from build123d import *

# Parameters (mm, degrees)
EXTRUDE_1_DEPTH          = 32
SKETCH_3_R               = 40
CUT_EXTRUDE_1_DEPTH      = 12
SKETCH_4_R               = 32.5
CUT_EXTRUDE_2_DEPTH      = 113
SKETCH_5_R               = 23.5
CUT_EXTRUDE_3_DEPTH      = 13
SKETCH_6_R               = 21
CUT_EXTRUDE_4_DEPTH      = 113
SKETCH_7_R               = 22.5
CUT_EXTRUDE_5_DEPTH      = 40
SKETCH_8_R               = 41.5
CUT_EXTRUDE_6_DEPTH      = 5.5
SKETCH_9_R               = 31
CUT_EXTRUDE_7_DEPTH      = 10
SKETCH_10_R              = 2.5
CUT_EXTRUDE_8_DEPTH      = 18
PATTERN_CIRCULAR_1_COUNT = 4
SKETCH_12_W              = 185
SKETCH_12_H              = 5
CUT_EXTRUDE_10_DEPTH     = 114
SKETCH_13_R              = 6
CUT_EXTRUDE_11_DEPTH     = 14
SKETCH_14_R              = 4
SKETCH_14_R_2            = 4.76
CUT_EXTRUDE_12_DEPTH     = 96
SKETCH_15_R              = 7
CUT_EXTRUDE_13_DEPTH     = 9
SKETCH_16_R              = 2.531047244
SKETCH_16_R_2            = 3
CUT_EXTRUDE_14_DEPTH     = 10
SKETCH_17_R              = 2.5
CUT_EXTRUDE_15_DEPTH     = 8


with BuildPart() as part:
    # 草图1 → 凸台-拉伸1 (new body)
    with BuildSketch(Plane.XY):
        Polygon((105, -80), (105, -6), (150, -6), (150, 147), (-30, 147), (-80, 97), (-80, -80), align=None)
    extrude(amount=EXTRUDE_1_DEPTH)

    # 草图3 → 切除-拉伸1 (cut)
    with BuildSketch(Plane.XY.offset(32)):
        Circle(SKETCH_3_R)
    extrude(amount=-CUT_EXTRUDE_1_DEPTH, mode=Mode.SUBTRACT)

    # 草图4 → 切除-拉伸2 (cut)
    with BuildSketch(Plane.XY.offset(20)):
        Circle(SKETCH_4_R)
    extrude(amount=-CUT_EXTRUDE_2_DEPTH, mode=Mode.SUBTRACT)

    # 草图5 → 切除-拉伸3 (cut)
    with BuildSketch(Plane(origin=(0, 0, 0), x_dir=(-1, 0, 0), z_dir=(0, 0, -1))):
        with Locations((0, 85)):
            Circle(SKETCH_5_R)
    extrude(amount=-CUT_EXTRUDE_3_DEPTH, mode=Mode.SUBTRACT)

    # 草图6 → 切除-拉伸4 (cut)
    with BuildSketch(Plane(origin=(0, 0, 13), x_dir=(-1, 0, 0), z_dir=(0, 0, -1))):
        with Locations((0, 85)):
            Circle(SKETCH_6_R)
    extrude(amount=-CUT_EXTRUDE_4_DEPTH, mode=Mode.SUBTRACT)

    # 草图7 → 切除-拉伸5 (cut)
    with BuildSketch(Plane(origin=(0, 0, 0), x_dir=(-1, 0, 0), z_dir=(0, 0, -1))):
        with Locations((-80, 85)):
            Circle(SKETCH_7_R)
    extrude(amount=-CUT_EXTRUDE_5_DEPTH, mode=Mode.SUBTRACT)

    # 草图8 → 切除-拉伸6 (cut)
    with BuildSketch(Plane.XY.offset(32)):
        with Locations((80, 85)):
            Circle(SKETCH_8_R)
    extrude(amount=-CUT_EXTRUDE_6_DEPTH, mode=Mode.SUBTRACT)

    # 草图9 → 切除-拉伸7 (cut)
    with BuildSketch(Plane(origin=(0, 0, 0), x_dir=(-1, 0, 0), z_dir=(0, 0, -1))):
        with Locations((-80, 85)):
            Circle(SKETCH_9_R)
    extrude(amount=-CUT_EXTRUDE_7_DEPTH, mode=Mode.SUBTRACT)

    # 草图10 → 切除-拉伸8 (cut)
    with BuildSketch(Plane(origin=(0, 0, 0), x_dir=(-1, 0, 0), z_dir=(0, 0, -1))):
        with Locations((-41, 85)):
            Circle(SKETCH_10_R)
    cut_extrude_8 = extrude(amount=-CUT_EXTRUDE_8_DEPTH, mode=Mode.SUBTRACT)

    # 阵列(圆周)1: 切除-拉伸8 ×4 about axis
    pattern_circular_1_axis = Axis((80, 85, 0), (0, 0, 1))
    for i in range(1, PATTERN_CIRCULAR_1_COUNT):
        add(cut_extrude_8.rotate(pattern_circular_1_axis, i * 360 / PATTERN_CIRCULAR_1_COUNT), mode=Mode.SUBTRACT)

    # 草图12 → 切除-拉伸10 (cut)
    with BuildSketch(Plane(origin=(0, 0, 0), x_dir=(-1, 0, 0), z_dir=(0, 0, -1))):
        with Locations((-12.5, -77.5)):
            Rectangle(SKETCH_12_W, SKETCH_12_H)
    extrude(amount=-CUT_EXTRUDE_10_DEPTH, mode=Mode.SUBTRACT)

    # 草图13 → 切除-拉伸11 (cut)
    with BuildSketch(Plane.XY.offset(32)):
        with Locations((80, 34)):
            Circle(SKETCH_13_R)
        with Locations((80, 136)):
            Circle(SKETCH_13_R)
    extrude(amount=-CUT_EXTRUDE_11_DEPTH, mode=Mode.SUBTRACT)

    # 草图14 → 切除-拉伸12 (cut)
    with BuildSketch(Plane.XY.offset(32)):
        with Locations((140, 137)):
            Circle(SKETCH_14_R)
        with Locations((140, 4)):
            Circle(SKETCH_14_R_2)
        with Locations((32, 137)):
            Circle(SKETCH_14_R_2)
        with Locations((-70, -65)):
            Circle(SKETCH_14_R)
        with Locations((95, -65)):
            Circle(SKETCH_14_R)
        with Locations((-70, 87)):
            Circle(SKETCH_14_R)
    extrude(amount=-CUT_EXTRUDE_12_DEPTH, mode=Mode.SUBTRACT)

    # 草图15 → 切除-拉伸13 (cut)
    with BuildSketch(Plane.XY.offset(32)):
        with Locations((140, 137)):
            Circle(SKETCH_15_R)
        with Locations((95, -65)):
            Circle(SKETCH_15_R)
        with Locations((-70, -65)):
            Circle(SKETCH_15_R)
        with Locations((-70, 87)):
            Circle(SKETCH_15_R)
    extrude(amount=-CUT_EXTRUDE_13_DEPTH, mode=Mode.SUBTRACT)

    # 草图16 → 切除-拉伸14 (cut)
    with BuildSketch(Plane.XY.offset(32)):
        with Locations((-44.393398282, 111.393398282)):
            Circle(SKETCH_16_R)
        with Locations((55, -60)):
            Circle(SKETCH_16_R_2)
        with Locations((-65, -25)):
            Circle(SKETCH_16_R_2)
        with Locations((15, 117)):
            Circle(SKETCH_16_R_2)
    extrude(amount=-CUT_EXTRUDE_14_DEPTH, mode=Mode.SUBTRACT)

    # 草图17 → 切除-拉伸15 (cut)
    with BuildSketch(Plane.XY.offset(32)):
        with Locations((-38, 30)):
            Circle(SKETCH_17_R)
        with Locations((-38, -30)):
            Circle(SKETCH_17_R)
    extrude(amount=-CUT_EXTRUDE_15_DEPTH, mode=Mode.SUBTRACT)


solid = part.part
The listing builds one solid part. Answer for the finished solid, in the listing's coordinates (mm). A direction names the side the tool comes from. Coordinates: 2 decimals unless noted, no trailing zeros. Loops run counter-clockwise (first coordinate to the right, second up) from the corner with the lowest first, then second, coordinate; pieces in that order, holes last. Notation, with made-up numbers: M 12,74 L 63,74 A25 cw 63,89 Z; hole C -25.5,32.25 d2. An arc over 180 degrees is marked long. Answer in a Markdown table with one row per item.
1) Given pin 1 (1.5 mm diameter, centred on x = 91, y = 11.5, fed in from -Z); pin 2 (4 mm diameter, centred on x = 96, y = -67.5, fed in from +Z); pin 3 (6.5 mm diameter, centred on x = -70, y = 87, fed in from -Z); pin 4 (1.5 mm diameter, centred on x = -43, z = 26.5, fed in from +Y), each flat-ended and moving along its own axis, determine where each tip first touches the part or whether it passes through.
Answers below:
| item | result |
|---|---|
| pin 1 | z = 0 |
| pin 2 | z = 23 |
| pin 3 | through |
| pin 4 | y = 134.75 |
2) Find section C-C (y = 21.5). Determine the outline of the cut face in (x, z), then the cut area to 3 significant figures.
Answers below:
| item | result |
|---|---|
| outline | M -80,0 L -24.37,0 L -24.37,20 L -33.73,20 L -33.73,32 L -80,32 Z; M 24.37,0 L 150,0 L 150,32 L 33.73,32 L 33.73,20 L 24.37,20 Z |
| area | 5,580 mm^2 |
3) Find the intervals of material crossed by probe 1 along X at (y, z) = (83.5, 19.5); probe 2 along Y at (x, z) = (15, 24); probe 3 along Y at (x, z) = (80, 23), in increasing order.
Answers below:
| item | result |
|---|---|
| probe 1 | -80 to -71.94, -68.06 to -20.95, 20.95 to 57.55, 102.45 to 150 |
| probe 2 | -75 to -37.08, 37.08 to 70.3, 99.7 to 114, 120 to 147 |
| probe 3 | -75 to 28, 40 to 62.5, 107.5 to 130, 142 to 147 |
4) Find section A-A (z = 7). Count the separate pieces of the cut face and the enclosed holes in it, then the cut area to 3 significant figures.
Answers below:
| item | result |
|---|---|
| separate pieces | 1 |
| enclosed holes | 13 |
| area | 38,200 mm^2 |
5) Determine the mould class of faces 4 (the cylindrical face through (-8.67, -39.05, 26.08)), 5 (the flat face through (105, -41, 16)), 6 (the flat face through (-55, 122, 16)) for opening direction Y: released by +Y, released by -Y, zero draft, split by the parting line, or undercut.
Answers below:
| item | result |
|---|---|
| face 4 | undercut |
| face 5 | zero draft |
| face 6 | released by +Y |
6) Find section B-B (x = 0). Determine the outline of the cut face in (y, z), then the cut area to 4 significant figures.
Answers below:
| item | result |
|---|---|
| outline | M -75,0 L -32.5,0 L -32.5,20 L -40,20 L -40,32 L -75,32 Z; M 32.5,0 L 61.5,0 L 61.5,13 L 64,13 L 64,32 L 40,32 L 40,20 L 32.5,20 Z; M 106,13 L 108.5,13 L 108.5,0 L 147,0 L 147,32 L 106,32 Z |
| area | 3,435 mm^2 |
7) Which of the six approach directions +Z, -Z, +X, -X, +Y, -Y give full straight-line access (tool end or side, diameter ignored) to faces 1 (the cylindrical face through (142.15, 140.373, 11.661)), 2 (the flat face through (119, 85, 18)), 3 (the cylindrical face through (15, 120, 27))?
Answers below:
| item | result |
|---|---|
| face 1 | +Z, -Z |
| face 2 | -Z |
| face 3 | +Z |
